For this review, take the finished solid that the model builds, in its own axes (mm). Face numbers are marked on the shaded views. Give positions to 0.01 mm unless a question says otherwise; leave off trailing zeros. Loops run counter-clockwise (first coordinate to the right, second up) from the corner with the lowest first, then second, coordinate; pieces in that order, holes last.
```python
from build123d import *

# Parameters (mm, degrees)
BOSS_EXTRUDE1_DEPTH = 64
BOSS_EXTRUDE2_DEPTH = 4
SKETCH4_W           = 54
SKETCH4_H           = 69
CUT_EXTRUDE1_DEPTH  = 5


with BuildPart() as part:
    # Sketch1 → Boss-Extrude1 (new body)
    with BuildSketch(Plane.XY):
        Polygon((0, 0), (7.5, 0), (-23.773751369, 67.066776241), (-26.927291044, 61.861401656), (-24.579993125, 52.711965363), align=None)
    extrude(amount=-BOSS_EXTRUDE1_DEPTH)

    # Sketch3 → Boss-Extrude2 (add)
    with BuildSketch(Plane(origin=(-10.373887242, -2.661432153, 0), x_dir=(0, 0, 1), z_dir=(-0.9686310353512481, -0.24850335481511932, 0))):
        Polygon((-36, 57.166656338), (-32, 57.166656338), (-28, 57.166656338), (-28, 60.166656338), (-36, 60.166656338), align=None)
    extrude(amount=BOSS_EXTRUDE2_DEPTH)

    # Sketch4 → Cut-Extrude1 (cut)
    with BuildSketch(Plane(origin=(6.160453536, 2.872666662, 0), x_dir=(0, 0, -1), z_dir=(0.9063077870366478, 0.4226182617407043, 0))):
        with Locations((32, 36.330363037)):
            Rectangle(SKETCH4_W, SKETCH4_H)
    extrude(amount=-CUT_EXTRUDE1_DEPTH, mode=Mode.SUBTRACT)


solid = part.part
```
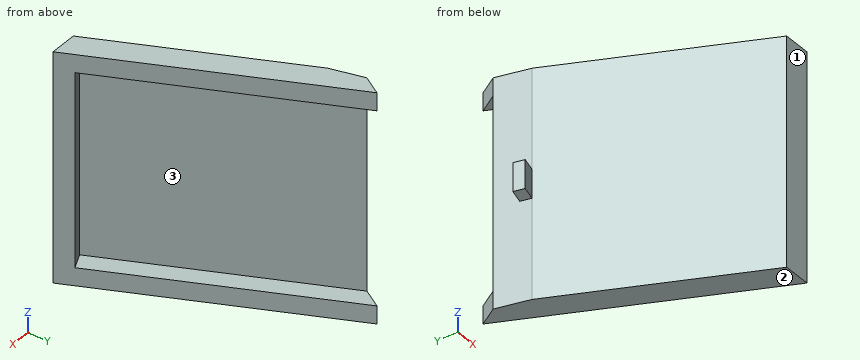
Q1. Mouldability with a two-part tool opening along Z and no side actions: class the marked faces 1, 2 and 3 as +Z half, -Z half, draft (parallel to the pull), parting line (faces both ways), or undercut.
Answers:
face 1: draft
face 2: -Z half
face 3: undercut
Q2. Consider section C-C on x = -1. Give the boundary of the cut face in (y, z), plus the area to 3 significant figures.
Answers:
outline: (2.14, -64) - (18.23, -64) - (18.23, -59) - (6.4, -59) - (6.4, -5) - (18.23, -5) - (18.23, 0) - (2.14, 0) - close
area: 390 mm2
Q3. For probe 1 along Z at (x, y) = (-20, 48.5); probe 2 along X at (y, z) = (59, -4.5); probe 3 along X at (y, z) = (8.5, -48), list the stretches that pass through material, from the lowest coordinate up.
Answers:
probe 1: z = -64 to -59, -5 to 0
probe 2: x = -26.19 to -20.01
probe 3: x = -3.96 to -1.98
Q4. Consider section D-D on z = -41.5. Give the boundary of the cut face in (x, y), plus the area to 3 significant figures.
Answers:
outline: (-26.93, 61.86) - (-24.58, 52.71) - (0, 0) - (7.5, 0) - (5.39, 4.53) - (0.86, 2.42) - (-26.89, 61.92) - close
area: 133 mm2
Q5. For pin 1 Ø12 at (y, z) = (40, -39.5) entering from -X; pin 2 Ø12 at (x, z) = (2, -40.5) entering from -Y; pin 3 Ø1.2 at (x, y) = (-26.5, 53.5) entering from -Z; pin 4 Ø3 at (x, y) = (-27.5, 54) entering from +Z, all flat-tipped, find the tip position at first contact; note any pin that passes through.
Answers:
pin 1: stops at x = -21.45
pin 2: stops at y = 0
pin 3: stops at z = -36
pin 4: stops at z = -28
Q6. Consider section B-B on y = 42. Give the boundary of the cut face in (x, z), plus the area to 3 significant figures.
Answers:
outline: (-19.58, -64) - (-12.08, -64) - (-12.08, -59) - (-17.6, -59) - (-17.6, -5) - (-12.08, -5) - (-12.08, 0) - (-19.58, 0) - close
area: 182 mm2
Q7. Consider section A-A on z = -34.5. Give the boundary of the cut face in (x, y).
Answers:
outline: (-29.2, 54.62) - (-28.45, 51.72) - (-24.58, 52.71) - (0, 0) - (7.5, 0) - (5.39, 4.53) - (0.86, 2.42) - (-26.89, 61.92) - (-26.93, 61.86) - (-25.33, 55.62) - close
